The listing builds one solid part. Answer for the finished solid, in the listing's coordinates (mm). Face numbers are marked on the shaded views. A direction names the side the tool comes from. Round coordinates to 2 decimals unless told otherwise and drop trailing zeros. Write each loop counter-clockwise with the first axis right and the second up, starting at its lowest first coordinate (ties: lowest second). Pieces come first, ordered by that corner, then holes.
Item 1: Each of these flat-tipped pins is pushed along its axis until it touches: pin 1 (1.2 mm diameter, centred on y = -29.5, z = 14, fed in from +X); pin 2 (8 mm diameter, centred on x = 0.5, y = -5, fed in from -Z); pin 3 (1.1 mm diameter, centred on y = 31, z = 4.5, fed in from +X). Where does it stop, or does it pass through?
Item 2: Find section B-B on z = 0. Give the vertices of the cut face in (x, y).
Item 3: Find the intervals of material crossed by probe 1 along X at (y, z) = (-46, -10.25); probe 2 along Z at (x, y) = (0, 20.5); probe 3 along X at (y, z) = (-46, -6.25), in increasing order.
Item 4: Find section A-A on x = 0. Give the vertices of the cut face in (y, z), then the cut area to 3 significant figures.
Item 5: For a pull along X with two mould halves and no side action, classify the marked faces 4 and 5 as +X half, -X half, draft (parallel to the pull), parting line (faces both ways), or undercut.
Item 6: Find section C-C on x = -7. Give the vertices of the cut face in (y, z), then the cut area to 3 significant figures.
Item 7: A tool of negligible diameter and unlimited length cuts with its end or side. For the marked faces 1, 2 and 3, from which of +Z, -Z, +X, -X, +Y, -Y can it reach the whole face along a straight path? Write none if from no direction.
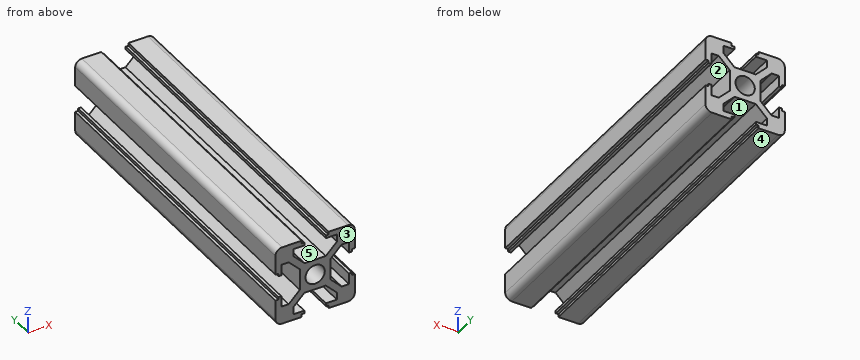
```python
from build123d import *

# Parameters (mm, degrees)
SKETCH13_R                          = 3.65
BOSCHREXROTH_BOSCH_30X30_V2_1_DEPTH = 127


with BuildPart() as part:
    # Sketch13 → Boschrexroth BOSCH_30X30_V2(1) (new body)
    with BuildSketch(Plane.XZ.offset(-63.5)):
        with BuildLine():
            Line((0, 5.8), (-4.03, 5.8))
            Line((-4.03, 5.8), (-8.25, 10.02))
            Line((-8.25, 10.02), (-8.25, 12.8))
            Line((-8.25, 12.8), (-4.1, 12.8))
            Line((-4.1, 12.8), (-4.1, 13.9))
            Line((-4.1, 13.9), (-5.1, 13.9))
            Line((-5.1, 13.9), (-5.1, 15))
            Line((-5.1, 15), (-12.5, 15))
            ThreePointArc((-12.5, 15), (-14.267766953, 14.267766953), (-15, 12.5))
            Line((-15, 12.5), (-15, 5.1))
            Line((-15, 5.1), (-13.9, 5.1))
            Line((-13.9, 5.1), (-13.9, 4.1))
            Line((-13.9, 4.1), (-12.8, 4.1))
            Line((-12.8, 4.1), (-12.8, 8.25))
            Line((-12.8, 8.25), (-10.02, 8.25))
            Line((-10.02, 8.25), (-5.8, 4.03))
            Line((-5.8, 4.03), (-5.8, 0))
            Line((-5.8, 0), (-5.8, -4.03))
            Line((-5.8, -4.03), (-10.02, -8.25))
            Line((-10.02, -8.25), (-12.8, -8.25))
            Line((-12.8, -8.25), (-12.8, -4.1))
            Line((-12.8, -4.1), (-13.9, -4.1))
            Line((-13.9, -4.1), (-13.9, -5.1))
            Line((-13.9, -5.1), (-15, -5.1))
            Line((-15, -5.1), (-15, -12.5))
            ThreePointArc((-15, -12.5), (-14.267766953, -14.267766953), (-12.5, -15))
            Line((-12.5, -15), (-5.1, -15))
            Line((-5.1, -15), (-5.1, -13.9))
            Line((-5.1, -13.9), (-4.1, -13.9))
            Line((-4.1, -13.9), (-4.1, -12.8))
            Line((-4.1, -12.8), (-8.25, -12.8))
            Line((-8.25, -12.8), (-8.25, -10.02))
            Line((-8.25, -10.02), (-4.03, -5.8))
            Line((-4.03, -5.8), (4.03, -5.8))
            Line((4.03, -5.8), (8.25, -10.02))
            Line((8.25, -10.02), (8.25, -12.8))
            Line((8.25, -12.8), (4.1, -12.8))
            Line((4.1, -12.8), (4.1, -13.9))
            Line((4.1, -13.9), (5.1, -13.9))
            Line((5.1, -13.9), (5.1, -15))
            Line((5.1, -15), (12.5, -15))
            ThreePointArc((12.5, -15), (14.267766953, -14.267766953), (15, -12.5))
            Line((15, -12.5), (15, -5.1))
            Line((15, -5.1), (13.9, -5.1))
            Line((13.9, -5.1), (13.9, -4.1))
            Line((13.9, -4.1), (12.8, -4.1))
            Line((12.8, -4.1), (12.8, -8.25))
            Line((12.8, -8.25), (10.02, -8.25))
            Line((10.02, -8.25), (5.8, -4.03))
            Line((5.8, -4.03), (5.8, 0))
            Line((5.8, 0), (5.8, 4.03))
            Line((5.8, 4.03), (10.02, 8.25))
            Line((10.02, 8.25), (12.8, 8.25))
            Line((12.8, 8.25), (12.8, 4.1))
            Line((12.8, 4.1), (13.9, 4.1))
            Line((13.9, 4.1), (13.9, 5.1))
            Line((13.9, 5.1), (15, 5.1))
            Line((15, 5.1), (15, 12.5))
            ThreePointArc((15, 12.5), (14.267766953, 14.267766953), (12.5, 15))
            Line((12.5, 15), (5.1, 15))
            Line((5.1, 15), (5.1, 13.9))
            Line((5.1, 13.9), (4.1, 13.9))
            Line((4.1, 13.9), (4.1, 12.8))
            Line((4.1, 12.8), (8.25, 12.8))
            Line((8.25, 12.8), (8.25, 10.02))
            Line((8.25, 10.02), (4.03, 5.8))
            Line((4.03, 5.8), (0, 5.8))
        make_face()
        Circle(SKETCH13_R, mode=Mode.SUBTRACT)
    extrude(amount=BOSCHREXROTH_BOSCH_30X30_V2_1_DEPTH)


solid = part.part
```
Check values:
1. pin 1: stops at x = 14.83
1. pin 2: stops at z = -13.9
1. pin 3: stops at x = 13.9
2. outline: (-5.8, -63.5) - (-3.65, -63.5) - (-3.65, 63.5) - (-5.8, 63.5) - close; (3.65, -63.5) - (5.8, -63.5) - (5.8, 63.5) - (3.65, 63.5) - close
3. probe 1: x = -15 to -8.25, 8.25 to 15
3. probe 2: z = -5.8 to -3.65, 3.65 to 5.8
3. probe 3: x = -15 to -12.8, -8.02 to -4.48, 4.48 to 8.02, 12.8 to 15
4. outline: (-63.5, -5.8) - (63.5, -5.8) - (63.5, -3.65) - (-63.5, -3.65) - close; (-63.5, 3.65) - (63.5, 3.65) - (63.5, 5.8) - (-63.5, 5.8) - close
4. area: 546 mm2
5. face 4: draft
5. face 5: undercut
6. outline: (-63.5, -15) - (63.5, -15) - (63.5, -12.8) - (-63.5, -12.8) - close; (-63.5, -8.77) - (63.5, -8.77) - (63.5, -5.23) - (-63.5, -5.23) - close; (-63.5, 5.23) - (63.5, 5.23) - (63.5, 8.77) - (-63.5, 8.77) - close; (-63.5, 12.8) - (63.5, 12.8) - (63.5, 15) - (-63.5, 15) - close
6. area: 1,460 mm2
7. face 1: -Z, +Y, -Y
7. face 2: +Y, -Y
7. face 3: +Z, -Z, +X, -X, -Y
